from build123d import *
from OCP.BRepAlgoAPI import BRepAlgoAPI_Cut
from OCP.TopTools import TopTools_ListOfShape

# Parameters (mm, degrees)
BOSS_EXTRUDE1_DEPTH      = 5.73
BOSS_EXTRUDE1_DEPTH_BACK = 5.73
BOSS_EXTRUDE5_DEPTH      = 11.46
BOSS_EXTRUDE8_DEPTH      = 11.46
BOSS_EXTRUDE9_DEPTH      = 3
SKETCH11_R               = 3.54
CUT_EXTRUDE1_DEPTH       = 3
BOSS_EXTRUDE10_DEPTH     = 3
SKETCH13_R               = 1.5
CUT_EXTRUDE2_DEPTH       = 3


with BuildPart() as part:
    # Sketch1 → Boss-Extrude1 (new, two sides: drawn at the far end of the back side and taken through both)
    with BuildSketch(Plane.XY.offset(-BOSS_EXTRUDE1_DEPTH_BACK)):
        Polygon((23.736099909, 38.996836219), (26.736100401, 35.996833865), (26.736100401, 3.776835326), (23.736098978, 0.776835766), (20.736098486, 3.77683812), (23.736098978, 6.776836749), (23.736098978, 32.99683803), (20.736100349, 35.996838521), align=None)
    extrude(amount=BOSS_EXTRUDE1_DEPTH + BOSS_EXTRUDE1_DEPTH_BACK)

    # Sketch6 → Boss-Extrude5 (add)
    with BuildSketch(Plane.XY.offset(5.73)):
        Polygon((20.736098486, 3.77683812), (8.576098486, 3.77683812), (8.576098486, 0.776835766), (20.736098486, 0.776835766), (23.736098978, 0.776835766), align=None)
    extrude(amount=-BOSS_EXTRUDE5_DEPTH)

    # Sketch8 → Boss-Extrude8 (add)
    with BuildSketch(Plane.XY.offset(5.73)):
        Polygon((20.736100349, 38.996836219), (23.736099909, 38.996836219), (20.736100349, 35.996838521), (8.576100349, 35.996838521), (8.576100349, 38.996836219), align=None)
    extrude(amount=-BOSS_EXTRUDE8_DEPTH)

    # Sketch9 → Boss-Extrude9 (add)
    with BuildSketch(Plane(origin=(0, 38.996836219, 0), x_dir=(1, 0, 0), z_dir=(0, 1, 0))):
        with BuildLine():
            Line((8.576100349, 5.73), (8.576100349, -5.73))
            ThreePointArc((8.576100349, -5.73), (-3.635159989, 0), (8.576100349, 5.73))
        make_face()
    extrude(amount=-BOSS_EXTRUDE9_DEPTH)

    # Sketch11 → Cut-Extrude1 (cut)
    with BuildSketch(Plane(origin=(0, 38.996836219, 0), x_dir=(1, 0, 0), z_dir=(0, 1, 0))):
        with Locations(Location((3.814840011, 0, 0), (0, 0, 270))):
            Circle(SKETCH11_R)
    extrude(amount=-CUT_EXTRUDE1_DEPTH, mode=Mode.SUBTRACT)

    # Sketch12 → Boss-Extrude10 (add)
    with BuildSketch(Plane(origin=(0, 0.776835766, 0), x_dir=(-1, 0, 0), z_dir=(0, -1, 0))):
        with BuildLine():
            Line((-8.576098486, 5.73), (-3.793078174, 5.73))
            ThreePointArc((-3.793078174, 5.73), (1.936921826, 0), (-3.793078174, -5.73))
            Line((-3.793078174, -5.73), (-8.576098486, -5.73))
            Line((-8.576098486, -5.73), (-8.576098486, 5.73))
        make_face()
    extrude(amount=-BOSS_EXTRUDE10_DEPTH)


with BuildPart() as cut_extrude2_tool:
    # Sketch13 → Cut-Extrude2 (new body)
    with BuildSketch(Plane(origin=(0, 3.77683812, 0), x_dir=(1, 0, 0), z_dir=(0, 1, 0))):
        with Locations(Location((3.81, 0, 0), (0, 0, 180))):
            Circle(SKETCH13_R)
    extrude(amount=-CUT_EXTRUDE2_DEPTH)


with BuildPart() as part_1:
    add(part.part)

    # Cut-Extrude2: cut by cut_extrude2_tool, with a tolerance
    cut_extrude2_stock = TopTools_ListOfShape()
    cut_extrude2_stock.Append(part_1.part.wrapped)
    cut_extrude2_tools = TopTools_ListOfShape()
    cut_extrude2_tools.Append(cut_extrude2_tool.part.wrapped)
    cut_extrude2_cut = BRepAlgoAPI_Cut()
    cut_extrude2_cut.SetArguments(cut_extrude2_stock)
    cut_extrude2_cut.SetTools(cut_extrude2_tools)
    cut_extrude2_cut.SetFuzzyValue(0.00001)
    cut_extrude2_cut.Build()
    add(Compound.cast(cut_extrude2_cut.Shape()).solids(), mode=Mode.REPLACE)


solid = part_1.part
Part model, mm, in its own coordinate system. A direction names the side the tool comes from. Coordinates: 2 decimals unless noted, no trailing zeros. Order: outer loops, then holes, each group sorted by start corner. A loop starts at its lowest first (then second) coordinate and runs counter-clockwise, first axis right, second up. Notation, with made-up numbers: M 56.25,31 L 88.25,31 A18 ccw 88.25,47 Z; hole C -3.5,-4.75 d3. An arc over 180 degrees is marked long. Use a Markdown table: item, result.
(1) Cut at D-D on y = 22. Write the cut outline in (x, z).
A:
| item | result |
|---|---|
| outline | M 23.74,-5.73 L 26.74,-5.73 L 26.74,5.73 L 23.74,5.73 Z |
(2) Pull direction X, two halves, no side cores. Call faces 1 (the cylindrical face through (-3.63, 37.52, 0.24)), 2 (the cylindrical face through (-1.936, 2.256, -0.126)), 3 (the flat face through (0, 35.997, 0)), 4 (the cylindrical face through (2.38, 2.3, 0.45)): released by +X, released by -X, zero draft, split by the parting line, or undercut.
A:
| item | result |
|---|---|
| face 1 | split by the parting line |
| face 2 | released by -X |
| face 3 | zero draft |
| face 4 | undercut |
(3) Probe L1, parallel to Y at x = 3, z = 3.5; L2, parallel to Z at x = 3.81, y = 1.95; L3, parallel to Y at x = 2, z = -1. List the from-to ranges inside material, lowest first.
A:
| item | result |
|---|---|
| L1 | y = 0.78 to 3.78, 36 to 39 |
| L2 | z = -5.73 to -1.5, 1.5 to 5.73 |
| L3 | y = 0.78 to 3.78 |
(4) Flat gauge pins, fed straight in: pin 1 (6 mm diameter, centred on x = 9, y = 31, fed in from +Z); pin 2 (4 mm diameter, centred on y = 25.5, z = -0.5, fed in from -X). Where does each tip first touch, or does it go through?
A:
| item | result |
|---|---|
| pin 1 | passes through |
| pin 2 | stops at x = 23.74 |
(5) Cut at B-B on x = 13.5. Write the cut outline in (y, z), then the cut area to 3 significant figures.
A:
| item | result |
|---|---|
| outline | M 0.78,-5.73 L 3.78,-5.73 L 3.78,5.73 L 0.78,5.73 Z; M 36,-5.73 L 39,-5.73 L 39,5.73 L 36,5.73 Z |
| area | 68.8 mm^2 |
(6) Cut at A-A on z = 0. State how many separate pieces and enclosed holes the cut face has, then the cut area to 3 significant figures.
A:
| item | result |
|---|---|
| separate pieces | 3 |
| enclosed holes | 0 |
| area | 244 mm^2 |
(7) Tool access for faces 5 (the flat face through (26.736, 20, 0)), 6 (the cylindrical face through (0.36, 37.52, -0.77)), 7 (the flat face through (15, 3.777, 0)): list every direction of +Z, -Z, +X, -X, +Y, -Y with a clear straight run to the whole face (end or side of a thin tool).
A:
| item | result |
|---|---|
| face 5 | +Z, -Z, +X, +Y, -Y |
| face 6 | +Y |
| face 7 | +Z, -Z, -X |
